Work out the finished part from the listing and answer in its coordinate system (mm). Coordinates: 2 decimals unless noted, no trailing zeros. Loops run counter-clockwise (first coordinate to the right, second up) from the corner with the lowest first, then second, coordinate; pieces in that order, holes last.
```python
from build123d import *

# Parameters (mm, degrees)
SKETCH1_R                   = 50.8
EXTRUDE1_DEPTH              = 25.4
F_1_4_0_25_DIAMETER_HOLE1_D = 6.35
F_1_4_20_TAPPED_HOLE1_D     = 5.1054
CIRPATTERN1_COUNT           = 4


with BuildPart() as part:
    # Sketch1 → Extrude1 (new body)
    with BuildSketch(Plane.XY):
        Circle(SKETCH1_R)
    extrude(amount=EXTRUDE1_DEPTH)

    # 1/4 (0.25) Diameter Hole1 (through all)
    with Locations(Plane.XY.offset(25.4)):
        with Locations((0, 0)):
            Hole(F_1_4_0_25_DIAMETER_HOLE1_D / 2)

    # 1/4-20 Tapped Hole1 (through all)
    with Locations(Plane(origin=(25.4, 0, 25.4), x_dir=(1, 0, 0), z_dir=(0, 0, 1))):
        with Locations((0, 0)):
            f_1_4_20_tapped_hole1 = Hole(F_1_4_20_TAPPED_HOLE1_D / 2)

    # CirPattern1: 1/4-20 Tapped Hole1 ×4 about axis
    cirpattern1_axis = Axis((0, 0, 0), (0, 0, 1))
    for i in range(1, CIRPATTERN1_COUNT):
        add(f_1_4_20_tapped_hole1.rotate(cirpattern1_axis, i * 360 / CIRPATTERN1_COUNT), mode=Mode.SUBTRACT)


solid = part.part
```
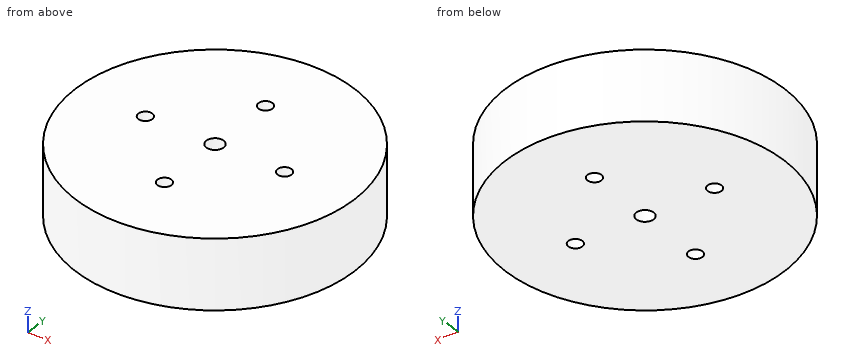
1. Each of these flat-tipped pins is pushed along its axis until it touches: P1, Ø3, axis at x = -30.5, z = 3.5, coming from the -Y side; P2, Ø12, axis at x = -17.5, z = 8.5, coming from the -Y side; P3, Ø10, axis at y = -33, z = 9.5, coming from the +X side. Where does it stop, or does it pass through?
2. A cutting plane is placed at C-C, the plane y = -25.4. Give the vertices of the cut face in (x, z).
3. A cutting plane is placed at A-A, the plane x = 0. Give the vertices of the cut face in (y, z) (3 decimals), then the cut area to 3 significant figures.
4. Straight lines are drawn through the part: probe 1 along Y at (x, z) = (-25.4, 5.75); probe 2 along X at (y, z) = (-24, 12.5); probe 3 along X at (y, z) = (34, 19). For each, find the intervals that lie inside material, in ascending order.
Answers below:
1. P1: stops at y = -41.71
1. P2: stops at y = -49.48
1. P3: stops at x = 42.39
2. outline: (-43.99, 0) - (-2.55, 0) - (-2.55, 25.4) - (-43.99, 25.4) - close; (2.55, 0) - (43.99, 0) - (43.99, 25.4) - (2.55, 25.4) - close
3. outline: (-50.8, 0) - (-27.953, 0) - (-27.953, 25.4) - (-50.8, 25.4) - close; (-22.847, 0) - (-3.175, 0) - (-3.175, 25.4) - (-22.847, 25.4) - close; (3.175, 0) - (22.847, 0) - (22.847, 25.4) - (3.175, 25.4) - close; (27.953, 0) - (50.8, 0) - (50.8, 25.4) - (27.953, 25.4) - close
3. area: 2,160 mm2
4. probe 1: y = -43.99 to -2.55, 2.55 to 43.99
4. probe 2: x = -44.77 to -2.13, 2.13 to 44.77
4. probe 3: x = -37.74 to 37.74
